Geometry check sheet. Reference: the model listing, model coordinates, mm. A direction names the side the tool comes from. Round coordinates to 2 decimals unless told otherwise and drop trailing zeros. Order: outer loops, then holes, each group sorted by start corner. A loop starts at its lowest first (then second) coordinate and runs counter-clockwise, first axis right, second up.
```python
from build123d import *

# Parameters (mm, degrees)
F0_W     = 3
F0_H     = 8
F0_H_2   = 3
F1_DEPTH = 40
F2_R     = 1


with BuildPart() as f1:
    # F0 (on Top) → F1 (new body)
    with BuildSketch(Plane.XY):
        with BuildLine():
            Line((-14.0882119191, 0), (0, 0))
            Line((0, 0), (0, 3))
            Line((0, 3), (-3, 3))
            Line((-3, 3), (-18, 3))
            Line((-18, 3), (-18, -5))
            Line((-18, -5), (-15, -5))
            Line((-15, -5), (-15, -0.87328878))
            Line((-15, -0.87328878), (-15.0993422135, -0.0114509659))
            ThreePointArc((-15.0993422135, -0.0114509659), (-15.0708824979, 0.0705384398), (-14.9890325392, 0.0993967545))
            Line((-14.9890325392, 0.0993967545), (-14.0882119191, 0))
        make_face()
        with Locations((-1.5, 7)):
            Rectangle(F0_W, F0_H)
        with Locations((1.5, 1.5)):
            Rectangle(F0_W, F0_H_2)
    extrude(amount=F1_DEPTH)

    # F2
    f2_edges = [f1.edges().sort_by_distance(p)[0] for p in [
        (-18, -5, 20),
        (-15, -5, 20),
        (-18, 3, 20),
        (3, 0, 20),
        (3, 3, 20),
        (-3, 3, 20),
        (-14.088212, 0, 20),
    ]]
    fillet(f2_edges, radius=F2_R)


solid = f1.part
```
(1) Sectioned sample at A-A, the plane z = 19.5. Record the cut outline in (x, y), and give its area (3 significant figures).
Returned:
outline: (-18, -4) arc R1 ccw to (-17, -5) - (-16, -5) arc R1 ccw to (-15, -4) - (-15, -0.87) - (-15.1, -0.01) arc R0.1 cw to (-14.99, 0.1) - (-14.14, 0.01) arc R1 ccw to (-14.03, 0) - (2, 0) arc R1 ccw to (3, 1) - (3, 2) arc R1 ccw to (2, 3) - (0, 3) - (0, 11) - (-3, 11) - (-3, 4) arc R1 cw to (-4, 3) - (-17, 3) arc R1 ccw to (-18, 2) - close
area: 101 mm2
(2) Draft check along X on faces 6 (the flat face through (-8, 1, 0)), 7 (the flat face through (-14.572, 0.053, 19.72)), 8 (the flat face through (0, 7, 20)), 9 (the cylindrical face through (-3.285, 3.301, 20.28)). Enter one of: released by +X, released by -X, zero draft, split by the parting line, or undercut.
Returned:
face 6: zero draft
face 7: undercut
face 8: released by +X
face 9: released by -X
(3) Material ranges on line 1 (X direction, y = -3.75, z = 17); line 2 (Y direction, x = 0.75, z = 37); line 3 (X direction, y = 10, z = 32), recorded low to high.
Returned:
line 1: x = -18 to -15
line 2: y = 0 to 3
line 3: x = -3 to 0
(4) Sectioned sample at C-C, the plane x = -1.5. Record the cut outline in (y, z), and give its area (3 significant figures).
Returned:
outline: (0, 0) - (11, 0) - (11, 40) - (0, 40) - close
area: 440 mm2
(5) Sectioned sample at B-B, the plane y = 8.5. Record the cut outline in (x, z), and give its area (3 significant figures).
Returned:
outline: (-3, 0) - (0, 0) - (0, 40) - (-3, 40) - close
area: 120 mm2
(6) Depth check by flat-ended pin: P1, Ø2.5, axis at y = 8.5, z = 22.5, coming from the +X side; P2, Ø1, axis at x = -6, z = 6, coming from the +Y side; P3, Ø8, axis at x = -9.5, z = 18.5, coming from the -Y side. Enter the tip coordinate at first touch or a pass-through.
Returned:
P1: stops at x = 0
P2: stops at y = 3
P3: stops at y = 0
(7) Set-up check for faces 1 (the flat face through (1, 3, 20)), 2 (the flat face through (-10, 3, 20)), 3 (the flat face through (-8, 1, 40)), 4 (the flat face through (-6, 0, 20)), 5 (the flat face through (-15.05, -0.45, 19.72)): record each of +Z, -Z, +X, -X, +Y, -Y from which the full face is reachable in a straight line by a thin tool's end or side.
Returned:
face 1: +Z, -Z, +X, +Y
face 2: +Z, -Z, -X, +Y
face 3: +Z, +X, -X, +Y, -Y
face 4: +Z, -Z, +X, -Y
face 5: +Z, -Z, +X
